For this review, take the finished solid that the model builds, in its own axes (mm). A direction names the side the tool comes from. Coordinates: 2 decimals unless noted, no trailing zeros. Loops run counter-clockwise (first coordinate to the right, second up) from the corner with the lowest first, then second, coordinate; pieces in that order, holes last. Notation, with made-up numbers: (6, 65) - (44, 65) arc R11 cw to (44, 69) - close; hole circle Ø1 at (-26, -34). An arc over 180 degrees is marked (long way). One line per item, written item: value. Start each with the question number.
1. Take a section at C-C, the plane x = 8.5. State the section outline as (y, z) points.
2. Take a section at D-D, the plane y = 5.5. State the section outline as (x, z) points, and give its area (3 significant figures).
3. Take a section at A-A, the plane z = 2. State the section outline as (x, y) points, and give its area (3 significant figures).
4. Insertion check: pin 1 (4 mm diameter, centred on x = 10.5, y = 10.5, fed in from +Z); pin 2 (5 mm diameter, centred on x = 19, y = 6.5, fed in from +Z); pin 3 (1.8 mm diameter, centred on x = -4.58, z = -36.5, fed in from -Y). Each pin has a flat end and moves straight along its axis. Give the tip position at first contact, or say it passes through.
5. To check wall thickness, follow line 1 (X direction, y = 33.5, z = -36.5); line 2 (X direction, y = 13.5, z = -35.5); line 3 (Z direction, x = 15, y = 9.5). State the ranges of each line that lie inside material, in increasing order. Write a range as from..to.
6. For faces 1 (the face through (-5.18, 0.57, 2.84)), 2 (the face through (-5.18, 20.25, 27.93)), 3 (the face through (10.18, 36.99, -14.35)), 4 (the face through (37.78, 39.4, 27.93)), list the 3-axis set-ups (+Z, -Z, +X, -X, +Y, -Y) from which the entire face can be reached by the end or side of a thin tool; tool diameter is ignored.
7. The part is to be moulded in two halves that separate along X. For faces 5 (the face through (11, 40, -28)), 6 (the face through (10.18, 2.85, -14.51)), 7 (the face through (-28.976, 0.57, -13.046)), 8 (the face through (49.85, 39.4, -10.97)), say which applies: released by +X, released by -X, zero draft, split by the parting line, or undercut.
8. Take a section at B-B, the plane y = 16. State the section outline as (x, z) points, and give its area (3 significant figures).
Autodesk Inventor part; units mm, degrees
ref_plane "YZ Plane" through (0, 0, 0) normal (1, 0, 0) x (0, 1, 0)
ref_plane "XZ Plane" through (0, 0, 0) normal (0, 1, 0) x (-1, 0, 0)
ref_plane "XY Plane" through (0, 0, 0) normal (0, 0, 1) x (1, 0, 0)
sketch "Эскиз1" plane through (0, 0, 0) normal (0, 1, 0) x (-1, 0, 0)
  line L0 (29.5774, -51.5004) -> (-50.4226, -51.5004)
  line L1 (-50.4226, -51.5004) -> (-50.4226, 28.4996)
  line L2 (-50.4226, 28.4996) -> (-25.4226, 28.4996)
  line L3 (-25.4226, 28.4996) -> (-25.4226, -11.5004)
  line L4 (-25.4226, -11.5004) -> (4.5774, -11.5004)
  line L5 (4.5774, -11.5004) -> (4.5774, 28.4996)
  line L6 (4.5774, 28.4996) -> (29.5774, 28.4996)
  line L7 (29.5774, 28.4996) -> (29.5774, -51.5004)
  point P0 (0, 0)
  dimension "d0" = 30
  dimension "d1" = 80
  dimension "d2" = 40
  dimension "d3" = 80
extrude "Выдавливание1" add sketch "Эскиз1" along normal blind 40
fillet "Сопряжение1" radius 10 2 edges at (10.4226, 40, -11.5004) (10.4226, 0, -11.5004)
fillet "Сопряжение2" radius 2 19 edges at (10.4226, 40, -51.5004) (-29.5774, 20, -51.5004) (50.4226, 20, -51.5004) (-17.0774, 40, 28.4996) (37.9226, 40, 28.4996) (37.9226, 0, 28.4996) (-17.0774, 0, 28.4996) (-4.5774, 40, 8.4996) (-29.5774, 40, -11.5004) (-29.5774, 0, -11.5004) (-29.5774, 20, 28.4996) (-4.5774, 20, 28.4996) (25.4226, 40, 8.4996) (25.4226, 20, 28.4996) (25.4226, 0, 8.4996) (-4.5774, 0, 8.4996) (50.4226, 20, 28.4996) (50.4226, 0, -11.5004) (50.4226, 40, -11.5004)
sketch "Эскиз2" plane through (0, 0, 0) normal (0, -1, 0) x (1, 0, 0)
  line L0 (-29.5774, 26.4996) -> (-29.5774, -49.5004)
  line L1 (-27.5774, -51.5004) -> (48.4226, -51.5004)
  point P0 (0, 0)
  point P1 (-4.5774, -36.5004)
  point P2 (25.4226, -36.5004)
  dimension "d8" = 30
  dimension "d9" = 25
  dimension "d10" = 15
hole "Отверстие1" at (-4.5774, 0, -36.5004) at (25.4226, 0, -36.5004) direction (0, 1, 0) diameter 3 end through all
properties part number "stand_holder"
Solutions:
1. outline: (0, -51.5) - (38, -51.5) arc R2 ccw to (40, -49.5) - (40, -21.5) arc R10 ccw to (30, -11.5) - (10, -11.5) arc R10 ccw to (0, -21.5) - close
2. outline: (-29.58, -49.5) arc R2 ccw to (-27.58, -51.5) - (48.42, -51.5) arc R2 ccw to (50.42, -49.5) - (50.42, 26.5) arc R2 ccw to (48.42, 28.5) - (27.42, 28.5) arc R2 ccw to (25.42, 26.5) - (25.42, -12.57) - (-4.58, -12.57) - (-4.58, 26.5) arc R2 ccw to (-6.58, 28.5) - (-27.58, 28.5) arc R2 ccw to (-29.58, 26.5) - close; hole circle Ø3 at (-4.58, -36.5); hole circle Ø3 at (25.42, -36.5)
2. area: 5,150 mm2
3. outline: (-29.58, 2) arc R2 ccw to (-27.58, 0) - (-6.58, 0) arc R2 ccw to (-4.58, 2) - (-4.58, 38) arc R2 ccw to (-6.58, 40) - (-27.58, 40) arc R2 ccw to (-29.58, 38) - close; (25.42, 2) arc R2 ccw to (27.42, 0) - (48.42, 0) arc R2 ccw to (50.42, 2) - (50.42, 38) arc R2 ccw to (48.42, 40) - (27.42, 40) arc R2 ccw to (25.42, 38) - close
3. area: 1,990 mm2
4. pin 1: z = -11.5
4. pin 2: z = -11.55
4. pin 3: through
5. line 1: -29.58..-6.08, -3.08..23.92, 26.92..50.42
5. line 2: -29.58..-5.7, -3.46..24.3, 26.54..50.42
5. line 3: -51.5..-11.51
6. face 1: +Z, -Y
6. face 2: +Z, +Y, -Y
6. face 3: +Z, +Y
6. face 4: +Z, +X, -X, +Y
7. face 5: zero draft
7. face 6: undercut
7. face 7: released by -X
7. face 8: released by +X
8. outline: (-29.58, -49.5) arc R2 ccw to (-27.58, -51.5) - (48.42, -51.5) arc R2 ccw to (50.42, -49.5) - (50.42, 26.5) arc R2 ccw to (48.42, 28.5) - (27.42, 28.5) arc R2 ccw to (25.42, 26.5) - (25.42, -11.5) - (-4.58, -11.5) - (-4.58, 26.5) arc R2 ccw to (-6.58, 28.5) - (-27.58, 28.5) arc R2 ccw to (-29.58, 26.5) - close; hole circle Ø3 at (-4.58, -36.5); hole circle Ø3 at (25.42, -36.5)
8. area: 5,180 mm2
